from build123d import *

# Parameters (mm, degrees)
CYLINDER_R        = 4.15
CYLINDER_DEPTH    = 3
CYLINDER001_R     = 6
CYLINDER001_DEPTH = 2
FILLET_R          = 1


with BuildPart() as cylinder:
    # Cylinder → Cylinder (new body)
    with BuildSketch(Plane.XY):
        Circle(CYLINDER_R)
    extrude(amount=CYLINDER_DEPTH)


with BuildPart() as cone:
    # Cone → Cone (revolve)
    with BuildSketch(Plane(origin=(0, 0, 3), x_dir=(1, 0, 0), z_dir=(0, -1, 0))):
        Polygon((0, 0), (4.15, 0), (3, 1), (0, 1), align=None)
    revolve(axis=Axis((0, 0, 3), (0, 0, 1)))


with BuildPart() as fusion:
    # Cylinder001 → Cylinder001 (new body)
    with BuildSketch(Plane.XY.offset(-2)):
        Circle(CYLINDER001_R)
    extrude(amount=CYLINDER001_DEPTH)

    # Fillet
    fillet_edges = [fusion.edges().sort_by_distance(p)[0] for p in [
        (-6, 0, -2),
    ]]
    fillet(fillet_edges, radius=FILLET_R)

    # Fusion: union Cylinder, Cone
    add(cylinder.part)
    add(cone.part)


solid = fusion.part
Work out the finished part from the listing and answer in its coordinate system (mm). A direction names the side the tool comes from. Give positions to 0.01 mm unless a question says otherwise; leave off trailing zeros. Loops run counter-clockwise (first coordinate to the right, second up) from the corner with the lowest first, then second, coordinate; pieces in that order, holes last. Notation, with made-up numbers: M -33.75,47.5 L -26.75,47.5 A14 ccw -26.75,54.5 Z; hole C -10,-2 d2. An arc over 180 degrees is marked long. Use CSV: the item, a comma, the result in double quotes.
1) Find section C-C on z = 1.25. Write down the section's boundary in (x, y), plus the area to 3 significant figures.
Answer:
outline,"C 0,0 d8.3"
area,"54.1 mm^2"
2) Consider L1, parallel to Z at x = 3.75, y = 3.25; L2, parallel to Y at x = 3.25, z = -1; L3, parallel to X at y = 4.75, z = -0.6. Determine where each line is inside the solid, lowest interval first.
Answer:
L1,"-2 to 0"
L2,"-5.04 to 5.04"
L3,"-3.67 to 3.67"
3) Find section A-A on y = 0. Write down the section's boundary in (x, z).
Answer:
outline,"M -6,-1 A1 ccw -5,-2 L 5,-2 A1 ccw 6,-1 L 6,0 L 4.15,0 L 4.15,3 L 3,4 L -3,4 L -4.15,3 L -4.15,0 L -6,0 Z"
4) Find section D-D on z = 3.55. Write down the section's boundary in (x, y) (1 decimal), plus the area to 3 significant figures.
Answer:
outline,"C 0,0 d7"
area,"38.9 mm^2"
5) Which of the six approach directions +Z, -Z, +X, -X, +Y, -Y give full straight-line access (tool end or side, diameter ignored) to faces 1 (the flat face through (0, 0, 4)), 2 (the flat face through (-4.1, 1.4, 0))?
Answer:
face 1,"+Z, +X, -X, +Y, -Y"
face 2,"+Z"
6) Given P1, Ø2, axis at x = 0, z = 3.5, coming from the -Y side; P2, Ø3, axis at y = 2.5, z = 0, coming from the +X side; P3, Ø6, axis at x = 3, y = -3, coming from the +Z side, each flat-ended and moving along its own axis, determine where each tip first touches the part or whether it passes through.
Answer:
P1,"y = -4.15"
P2,"x = 5.92"
P3,"z = 4"
